Can you work these out from the model? Positions are in its coordinate system, mm. Face numbers are marked on the shaded views. A direction names the side the tool comes from. Round coordinates to 2 decimals unless told otherwise and drop trailing zeros. Order: outer loops, then holes, each group sorted by start corner. A loop starts at its lowest first (then second) coordinate and runs counter-clockwise, first axis right, second up. Notation, with made-up numbers: (61.5, 81) -> (98.5, 81) arc R21 ccw to (98.5, 106) -> close; hole circle Ø2 at (48.5, 7). An arc over 180 degrees is marked (long way). Use a Markdown table: item, result. Add a question column.
Q1. If we section it at A-A on z = 0: List the corners of the cut face in (x, y) for me, plus the area to 3 significant figures.
Q2. I'm going to push flat-ended pins straight in: pin 1 Ø10.5 at (x, z) = (3, 4) entering from -Y; pin 2 Ø3 at (x, y) = (-6, -3) entering from +Z; pin 3 Ø1.5 at (y, z) = (-2, 2.5) entering from -X. Where does each tip first touch, or does it pass through?
Q3. If we section it at C-C on x = -5.5: List the corners of the cut face in (y, z) for me.
Q4. For the marked faces 1 and 2, which set-ups out of +Z, -Z, +X, -X, +Y, -Y let a thin tool reach every point of the face, with its end or its side?
Q5. We'd pull the mould along Z, two halves only. Please class the marked faces 3 and 4: +Z half, -Z half, draft (parallel to the pull), parting line (faces both ways), or undercut.
Q6. I need wall thicknesses on line 1 along Y through (x, z) = (2.25, 9); line 2 along Y through (x, z) = (-3, -10.5); line 3 along Z through (x, y) = (-5, -1.5). Which ranges of each line are inside material? Lowest first, please. Write a range as [from, to].
Q7. If we section it at D-D on z = -7: List the corners of the cut face in (x, y) for me, plus the area to 3 significant figures.
Q8. If we section it at B-B on y = -1.75: List the corners of the cut face in (x, z) for me, plus the area to 3 significant figures.
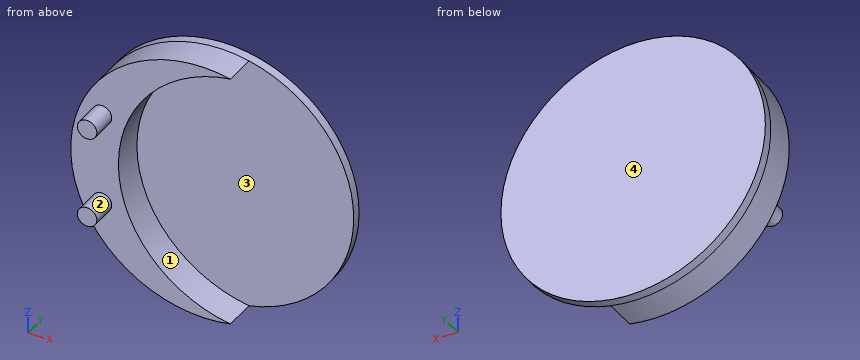
```python
from build123d import *

# Parameters (mm, degrees)
F0_R     = 12.9
F1_DEPTH = 0.9
F3_DEPTH = 3.1
F4_R     = 0.95
F5_DEPTH = 2.5


with BuildPart() as f1:
    # F0 (on Front) → F1 (new body)
    with BuildSketch(Plane.XZ):
        Circle(F0_R)
    extrude(amount=F1_DEPTH)

    # F2 (on face) → F3 (join)
    with BuildSketch(Plane.XZ.offset(0.9)):
        with BuildLine():
            ThreePointArc((2.6775, -12.619073), (-8.25, 0), (2.6775, 12.619073))
            ThreePointArc((2.6775, 12.619073), (-12.9, 0), (2.6775, -12.619073))
        make_face()
    extrude(amount=F3_DEPTH)

    # F4 (on face) → F5 (join)
    with BuildSketch(Plane.XZ.offset(4)):
        with Locations((-9.85, 4.5)):
            Circle(F4_R)
        with Locations((-9.85, -4.5)):
            Circle(F4_R)
    extrude(amount=F5_DEPTH)


solid = f1.part
```
Answer below:
| question | item | result |
|---|---|---|
| 1 | outline | (-12.9, -4) -> (-8.25, -4) -> (-8.25, -0.9) -> (12.9, -0.9) -> (12.9, 0) -> (-12.9, 0) -> close |
| 1 | area | 37.6 mm² |
| 2 | pin 1 | y = -0.9 |
| 2 | pin 2 | z = 12.09 |
| 2 | pin 3 | x = -12.78 |
| 3 | outline | (-4, -11.67) -> (0, -11.67) -> (0, 11.67) -> (-4, 11.67) -> (-4, 7.91) -> (-0.9, 7.91) -> (-0.9, -7.91) -> (-4, -7.91) -> close |
| 4 | face 1 | +X, -Y |
| 4 | face 2 | -Y |
| 5 | face 3 | undercut |
| 5 | face 4 | draft |
| 6 | line 1 | [-0.9, 0] |
| 6 | line 2 | [-4, 0] |
| 6 | line 3 | [-11.89, -8.5], [8.5, 11.89] |
| 7 | outline | (-10.84, -4) -> (-6.16, -4) -> (-6.16, -0.9) -> (10.84, -0.9) -> (10.84, 0) -> (-10.84, 0) -> close |
| 7 | area | 34.0 mm² |
| 8 | outline | (2.68, -12.62) arc R12.75 cw to (2.68, 12.62) arc R12.9 ccw (long way) to start |
| 8 | area | 121 mm² |
